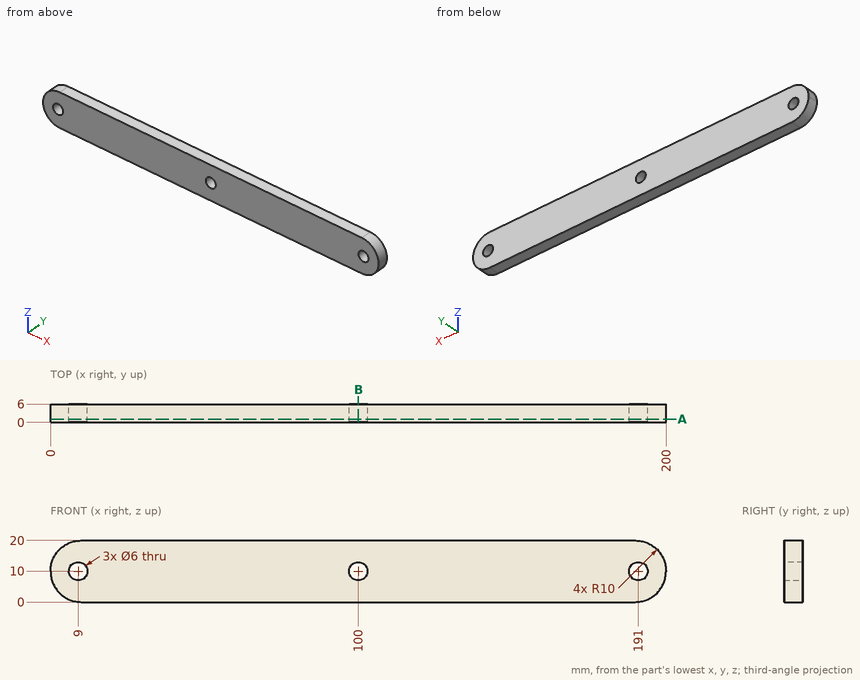
Design review of the part shown in the three views and the two pictorial views. Dimensions are in mm from the part's minimum x, y and z. Round coordinates to 2 decimals unless told otherwise and drop trailing zeros. Loops run counter-clockwise (first coordinate to the right, second up) from the corner with the lowest first, then second, coordinate; pieces in that order, holes last.
1) Wall thickness on line 1 along X through (y, z) = (2.6, 10); line 2 along X through (y, z) = (1.65, 8.5); line 3 along Z through (x, y) = (191, 3.9): over which ranges is each line inside the solid? List them lowest first.
Values follow:
line 1: x = 0 to 6, 12 to 97, 103 to 188, 194 to 200
line 2: x = 0.11 to 6.4, 11.6 to 97.4, 102.6 to 188.4, 193.6 to 199.89
line 3: z = 0.05 to 7, 13 to 19.95
2) Clearance check with a flat-ended pin moving along its axis: P1, Ø2, axis at y = 2.5, z = 4, coming from the +X side. State where the tip first meets the part, or that it passes through.
Values follow:
P1: stops at x = 198.66
3) Consider section B-B on x = 100. State the section outline as (y, z) points, then the cut area to 3 significant figures.
Values follow:
outline: (0, 0) - (6, 0) - (6, 7) - (0, 7) - close; (0, 13) - (6, 13) - (6, 20) - (0, 20) - close
area: 84.0 mm2
4) Consider section A-A on y = 1.1. Give the number of separate pieces and of enclosed holes in the cut face, then the cut area to 3 significant figures.
Values follow:
separate pieces: 1
enclosed holes: 3
area: 3,830 mm2
